Build history of the part. All positions in model axes, mm. A direction names the side the tool comes from. Round coordinates to 2 decimals unless told otherwise and drop trailing zeros. Write each loop counter-clockwise with the first axis right and the second up, starting at its lowest first coordinate (ties: lowest second). Pieces come first, ordered by that corner, then holes.
1) Saw through at A-A (x = 18.5). Write the cut outline in (y, z), plus the area to 3 significant figures.
2) Pull direction Z, two halves, no side cores. Call faces 5 (the flat face through (22, -7, -80)), 6 (the flat face through (24, -10, -55)), 7 (the flat face through (-56, 31, 0)): +Z half, -Z half, draft (parallel to the pull), parting line (faces both ways), or undercut.
3) Saw through at C-C (y = -7.5). Write the cut outline in (x, z).
4) Saw through at B-B (z = 15). Write the cut outline in (x, y), plus the area to 3 significant figures.
5) Saw through at D-D (x = -36). Write the cut outline in (y, z).
6) Wall check: probe 1 along Z at (x, y) = (9.5, -9); probe 2 along Y at (x, z) = (1.5, 56.5); probe 3 along X at (y, z) = (10, 8.5). Give the ranges that are in metal, low to high.
7) Flat gauge pins, fed straight in: pin 1 (4 mm diameter, centred on y = -5, z = 60, fed in from +X); pin 2 (4 mm diameter, centred on x = -26, z = 3.5, fed in from +Y); pin 3 (10 mm diameter, centred on x = -9.5, z = 23, fed in from +Y). Where does each tip first touch, or does it go through?
8) Which spindle directions (+Z, -Z, +X, -X, +Y, -Y) get a long thin tool onto all of the face, cutting with end or side? Do faces 1 (the flat face through (-6.7, 28.96, 0.35)), 2 (the flat face through (24, -5, -76)), 3 (the flat face through (22, 0, 1)), 4 (the flat face through (44, -12, -52)). Say none if no direction does.
from build123d import *

# Parameters (mm, degrees)
PAD_DEPTH    = 10
SKETCH001_W  = 10
SKETCH001_H  = 50
PAD001_DEPTH = 52
PAD002_DEPTH = 4
PAD003_DEPTH = 50


with BuildPart() as part:
    # Sketch → Pad (new body)
    with BuildSketch(Plane.XZ):
        Polygon((44, 76), (4, 76), (4, 35.5), (44, 35.5), (44, -35.5), (4, -35.5), (4, -76), (44, -76), (44, -80), (0, -80), (0, 80), (44, 80), align=None)
    extrude(amount=PAD_DEPTH)

    # Sketch001 (on Face14 of Pad) → Pad001 (join)
    with BuildSketch(Plane.XZ.offset(10)):
        with Locations((49, 0)):
            Rectangle(SKETCH001_W, SKETCH001_H)
    extrude(amount=-PAD001_DEPTH)

    # Sketch002 (on Face20 of Pad001) → Pad002 (join)
    with BuildSketch(Plane.XZ.offset(10)):
        Polygon((44, 80), (44, 25), (54, 25), (54, -25), (44, -25), (44, -80), (0, -80), (0, 80), align=None)
    extrude(amount=PAD002_DEPTH)

    # Sketch003 (on Face20 of Pad002) → Pad003 (join)
    with BuildSketch(Plane.XY.offset(25)):
        Polygon((44, 42), (-56, 36), (-56, 26), (44, 32), align=None)
    extrude(amount=-PAD003_DEPTH)


solid = part.part
Evaluation:
1. outline: (-14, -80) - (0, -80) - (0, -76) - (-10, -76) - (-10, -35.5) - (0, -35.5) - (0, 35.5) - (-10, 35.5) - (-10, 76) - (0, 76) - (0, 80) - (-14, 80) - close; (30.47, -25) - (40.47, -25) - (40.47, 25) - (30.47, 25) - close
1. area: 1,930 mm2
2. face 5: -Z half
2. face 6: undercut
2. face 7: draft
3. outline: (0, -80) - (44, -80) - (44, -76) - (4, -76) - (4, -35.5) - (44, -35.5) - (44, -25) - (54, -25) - (54, 25) - (44, 25) - (44, 35.5) - (4, 35.5) - (4, 76) - (44, 76) - (44, 80) - (0, 80) - close
4. outline: (-56, 26) - (44, 32) - (44, 0) - (0, 0) - (0, -14) - (54, -14) - (54, 42) - (44, 42) - (-56, 36) - close
4. area: 2,180 mm2
5. outline: (27.2, -25) - (37.2, -25) - (37.2, 25) - (27.2, 25) - close
6. probe 1: z = -80 to -76, -35.5 to 35.5, 76 to 80
6. probe 2: y = -14 to 0
6. probe 3: x = 44 to 54
7. pin 1: stops at x = 4
7. pin 2: stops at y = 37.92
7. pin 3: stops at y = 39.09
8. face 1: +Z, -Z
8. face 2: +X, +Y
8. face 3: +Z, -Z, -X
8. face 4: -Z, +X, +Y, -Y
